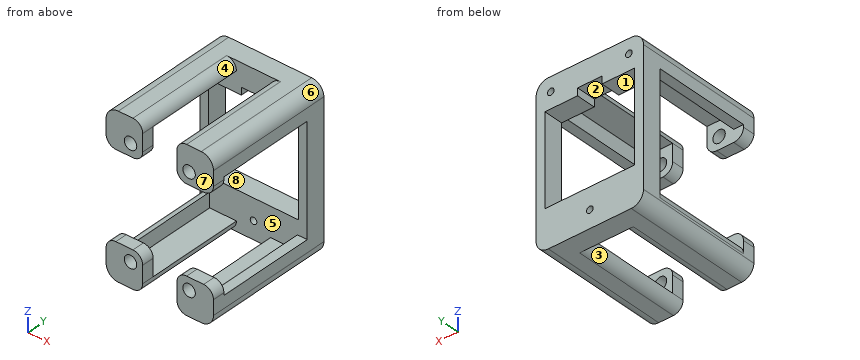
```python
from build123d import *

# Parameters (mm, degrees)
SKETCH1_W               = 44
SKETCH1_H               = 65
BOSS_EXTRUDE1_DEPTH     = 8
CUT_EXTRUDE1_REACH      = 42.053
SKETCH2_W               = 36.8
SKETCH2_H               = 36.8
CUT_EXTRUDE2_REACH      = 42.053
SKETCH3_R               = 1.35
BOSS_EXTRUDE2_DEPTH     = 40
SKETCH6_W               = 15
SKETCH6_H               = 15
BOSS_EXTRUDE3_DEPTH     = 5
CUT_EXTRUDE3_REACH      = 64.002
SKETCH7_R               = 2.55
MIRROR2_COPY_1_DEPTH    = 40
MIRROR2_COPY_2_SKETCH_W = 15
MIRROR2_COPY_2_SKETCH_H = 15
MIRROR2_COPY_2_DEPTH    = 5
MIRROR2_COPY_3_REACH    = 64.002
MIRROR2_COPY_3_SKETCH_R = 2.55
CUT_EXTRUDE4_REACH      = 67.949
SKETCH8_W               = 10
SKETCH8_H               = 3
FILLET1_R               = 4
FILLET2_R               = 5


with BuildPart() as part:
    # Sketch1 → Boss-Extrude1 (new body)
    with BuildSketch(Plane(origin=(0, 0, 0), x_dir=(1, 0, 0), z_dir=(0, 1, 0))):
        Rectangle(SKETCH1_W, SKETCH1_H)
    extrude(amount=BOSS_EXTRUDE1_DEPTH)

    # Sketch2 → Cut-Extrude1 (cut, up to next)
    with BuildSketch(Plane(origin=(0, 8, 0), x_dir=(1, 0, 0), z_dir=(0, 1, 0)), mode=Mode.PRIVATE) as cut_extrude1_sk1:
        with Locations((0, -1.8)):
            Rectangle(SKETCH2_W, SKETCH2_H)
    cut_extrude1_tool1 = extrude(cut_extrude1_sk1.sketch, amount=-CUT_EXTRUDE1_REACH, mode=Mode.PRIVATE) & part.part
    add(cut_extrude1_tool1.solids().sort_by_distance((0, 8, 1.8))[0], mode=Mode.SUBTRACT)

    # Sketch3 → Cut-Extrude2 (cut, up to next)
    with BuildSketch(Plane(origin=(0, 8, 0), x_dir=(1, 0, 0), z_dir=(0, 1, 0)), mode=Mode.PRIVATE) as cut_extrude2_sk1:
        with Locations(Location((-16, -26.7, 0), (0, 0, 270))):
            Circle(SKETCH3_R)
    cut_extrude2_tool1 = extrude(cut_extrude2_sk1.sketch, amount=-CUT_EXTRUDE2_REACH, mode=Mode.PRIVATE) & part.part
    # Sketch3 → Cut-Extrude2 (cut, up to next)
    with BuildSketch(Plane(origin=(0, 8, 0), x_dir=(1, 0, 0), z_dir=(0, 1, 0)), mode=Mode.PRIVATE) as cut_extrude2_sk2:
        with Locations(Location((16, -26.7, 0), (0, 0, 270))):
            Circle(SKETCH3_R)
    cut_extrude2_tool2 = extrude(cut_extrude2_sk2.sketch, amount=-CUT_EXTRUDE2_REACH, mode=Mode.PRIVATE) & part.part
    # Sketch3 → Cut-Extrude2 (cut, up to next)
    with BuildSketch(Plane(origin=(0, 8, 0), x_dir=(1, 0, 0), z_dir=(0, 1, 0)), mode=Mode.PRIVATE) as cut_extrude2_sk3:
        with Locations(Location((0, 25.3, 0), (0, 0, 270))):
            Circle(SKETCH3_R)
    cut_extrude2_tool3 = extrude(cut_extrude2_sk3.sketch, amount=-CUT_EXTRUDE2_REACH, mode=Mode.PRIVATE) & part.part
    add(cut_extrude2_tool1.solids().sort_by_distance((-16, 8, 26.7))[0], mode=Mode.SUBTRACT)
    add(cut_extrude2_tool2.solids().sort_by_distance((16, 8, 26.7))[0], mode=Mode.SUBTRACT)
    add(cut_extrude2_tool3.solids().sort_by_distance((0, 8, -25.3))[0], mode=Mode.SUBTRACT)

    # Sketch5 → Boss-Extrude2 (add)
    with BuildSketch(Plane.XZ):
        Polygon((22, 32.5), (7, 32.5), (7, 28.5), (18, 28.5), (18, 22.5), (22, 22.5), align=None)
    boss_extrude2 = extrude(amount=BOSS_EXTRUDE2_DEPTH)

    # Sketch6 → Boss-Extrude3 (add)
    with BuildSketch(Plane.XZ.offset(40)):
        with Locations((14.5, 25)):
            Rectangle(SKETCH6_W, SKETCH6_H)
    boss_extrude3 = extrude(amount=BOSS_EXTRUDE3_DEPTH)

    # Sketch7 → Cut-Extrude3 (cut, up to next)
    with BuildSketch(Plane(origin=(0, -40, 0), x_dir=(1, 0, 0), z_dir=(0, 1, 0)), mode=Mode.PRIVATE) as cut_extrude3_sk1:
        with Locations(Location((12, -22.5, 0), (0, 0, 270))):
            Circle(SKETCH7_R)
    cut_extrude3_tool1 = extrude(cut_extrude3_sk1.sketch, amount=-CUT_EXTRUDE3_REACH, mode=Mode.PRIVATE) & part.part
    cut_extrude3 = cut_extrude3_tool1.solids().sort_by_distance((12, -40, 22.5))[0]
    add(cut_extrude3, mode=Mode.SUBTRACT)

    # Mirror1: Boss-Extrude2, Boss-Extrude3, Cut-Extrude3 across plane
    add(boss_extrude2.mirror(Plane(origin=(0, 0, 0), x_dir=(0, 0, 1), z_dir=(1, 0, 0))))
    add(boss_extrude3.mirror(Plane(origin=(0, 0, 0), x_dir=(0, 0, 1), z_dir=(1, 0, 0))))
    add(cut_extrude3.mirror(Plane(origin=(0, 0, 0), x_dir=(0, 0, 1), z_dir=(1, 0, 0))), mode=Mode.SUBTRACT)

    # Mirror2: Boss-Extrude2, Boss-Extrude3, Cut-Extrude3 across plane
    add(boss_extrude2.mirror(Plane.XY))
    add(boss_extrude3.mirror(Plane.XY))
    add(cut_extrude3.mirror(Plane.XY), mode=Mode.SUBTRACT)

    # Mirror2 copy 1 sketch → Mirror2 copy 1 (add)
    with BuildSketch(Plane(origin=(0, 0, 0), x_dir=(-1, 0, 0), z_dir=(0, -1, 0))):
        Polygon((22, 32.5), (7, 32.5), (7, 28.5), (18, 28.5), (18, 22.5), (22, 22.5), align=None)
    extrude(amount=MIRROR2_COPY_1_DEPTH)

    # Mirror2 copy 2 sketch → Mirror2 copy 2 (add)
    with BuildSketch(Plane(origin=(0, -40, 0), x_dir=(-1, 0, 0), z_dir=(0, -1, 0))):
        with Locations((14.5, 25)):
            Rectangle(MIRROR2_COPY_2_SKETCH_W, MIRROR2_COPY_2_SKETCH_H)
    extrude(amount=MIRROR2_COPY_2_DEPTH)

    # Mirror2 copy 3 sketch → Mirror2 copy 3 (cut, up to next)
    with BuildSketch(Plane(origin=(0, -40, 0), x_dir=(-1, 0, 0), z_dir=(0, 1, 0)), mode=Mode.PRIVATE) as mirror2_copy_3_sk1:
        with Locations(Location((12, -22.5, 0), (0, 0, 270))):
            Circle(MIRROR2_COPY_3_SKETCH_R)
    mirror2_copy_3_tool1 = extrude(mirror2_copy_3_sk1.sketch, amount=-MIRROR2_COPY_3_REACH, mode=Mode.PRIVATE) & part.part
    add(mirror2_copy_3_tool1.solids().sort_by_distance((-12, -40, -22.5))[0], mode=Mode.SUBTRACT)

    # Sketch8 → Cut-Extrude4 (cut, up to next)
    with BuildSketch(Plane(origin=(0, 8, 0), x_dir=(1, 0, 0), z_dir=(0, 1, 0)), mode=Mode.PRIVATE) as cut_extrude4_sk1:
        with Locations((0, -21.7)):
            Rectangle(SKETCH8_W, SKETCH8_H)
    cut_extrude4_tool1 = extrude(cut_extrude4_sk1.sketch, amount=-CUT_EXTRUDE4_REACH, mode=Mode.PRIVATE) & part.part
    add(cut_extrude4_tool1.solids().sort_by_distance((0, 8, 21.7))[0], mode=Mode.SUBTRACT)

    # Fillet1
    fillet1_edges = [part.edges().sort_by_distance(p)[0] for p in [
        (7, -22.5, -32.5),
        (22, -42.5, -17.5),
        (7, -42.5, -17.5),
        (-22, -20, -22.5),
        (-7, -22.5, -32.5),
        (-22, -42.5, -17.5),
        (-7, -42.5, -17.5),
        (7, -22.5, 32.5),
        (22, -42.5, 17.5),
        (7, -42.5, 17.5),
        (-7, -22.5, 32.5),
        (-22, -42.5, 17.5),
        (-7, -42.5, 17.5),
    ]]
    fillet(fillet1_edges, radius=FILLET1_R - 0.0001)  # a hair under: the kernel refuses the full size

    # Fillet2
    fillet2_edges = [part.edges().sort_by_distance(p)[0] for p in [
        (-22, -18.5, -32.5),
        (22, -18.5, -32.5),
        (22, -18.5, 32.5),
        (-22, -18.5, 32.5),
    ]]
    fillet(fillet2_edges, radius=FILLET2_R)


solid = part.part
```
For this review, take the finished solid that the model builds, in its own axes (mm). Face numbers are marked on the shaded views. A direction names the side the tool comes from. Round coordinates to 2 decimals unless told otherwise and drop trailing zeros. Loops run counter-clockwise (first coordinate to the right, second up) from the corner with the lowest first, then second, coordinate; pieces in that order, holes last.
(1) Tool access review of the marked faces 1, 2, 3, 4 and 5: name each direction out of +Z, -Z, +X, -X, +Y, -Y from which nothing blocks a thin tool from reaching the whole face with its end or side.
Returned:
face 1: +Y
face 2: +Y, -Y
face 3: -Z, -Y
face 4: +Z, -Y
face 5: none
(2) We need section A-A (z = 16). Give the boundary of the cut face in (x, y), plus the area to 3 significant figures.
Returned:
outline: (-22, 0) - (-18.4, 0) - (-18.4, 8) - (-22, 8) - close; (18.4, 0) - (22, 0) - (22, 8) - (18.4, 8) - close
area: 57.6 mm2
(3) We need section C-C (y = -36.5). State how many separate pieces and enclosed holes the cut face has, plus the area to 3 significant figures.
Returned:
separate pieces: 4
enclosed holes: 0
area: 297 mm2
(4) Clearance check with flat-ended pins moving along their axes: P1, Ø4, axis at x = 8.5, y = -4, coming from the +Z side; P2, Ø12, axis at x = 9.5, z = 12.5, coming from the +Y side. State where each tip first meets the part, or that it passes through.
Returned:
P1: stops at z = 32.47
P2: stops at y = -40
(5) We need section D-D (z = 26.7). Give the boundary of the cut face in (x, y), plus the area to 3 significant figures.
Returned:
outline: (-22, -45) - (-7, -45) - (-7, -40) - (-18, -40) - (-18, 0) - (-17.35, 0) - (-17.35, 8) - (-22, 8) - close; (-14.65, 0) - (14.65, 0) - (14.65, 8) - (-14.65, 8) - close; (7, -45) - (22, -45) - (22, 8) - (17.35, 8) - (17.35, 0) - (18, 0) - (18, -40) - (7, -40) - close
area: 779 mm2
(6) Wall thickness on line 1 along X through (y, z) = (-42.15, 22.5); line 2 along Y through (x, z) = (17, -24); line 3 along X through (y, z) = (3.5, -25.3): over which ranges is each line inside the solid? List them lowest first.
Returned:
line 1: x = -22 to -14.55, -9.45 to -7, 7 to 9.45, 14.55 to 22
line 2: y = -45 to -40, 0 to 8
line 3: x = -22 to -1.35, 1.35 to 22
(7) We need section B-B (x = 16). Give the boundary of the cut face in (y, z), plus the area to 3 significant figures.
Returned:
outline: (-45, -32.5) - (8, -32.5) - (8, -16.6) - (0, -16.6) - (0, -28.5) - (-40, -28.5) - (-40, -17.5) - (-45, -17.5) - close; (-45, 17.5) - (-40, 17.5) - (-40, 28.5) - (0, 28.5) - (0, 28.05) - (8, 28.05) - (8, 32.5) - (-45, 32.5) - close; (0, 20.2) - (8, 20.2) - (8, 25.35) - (0, 25.35) - close
area: 674 mm2
(8) Mouldability with a two-part tool opening along Z and no side actions: class the marked faces 6, 7 and 8 as released by +Z, released by -Z, zero draft, split by the parting line, or undercut.
Returned:
face 6: released by +Z
face 7: zero draft
face 8: undercut
